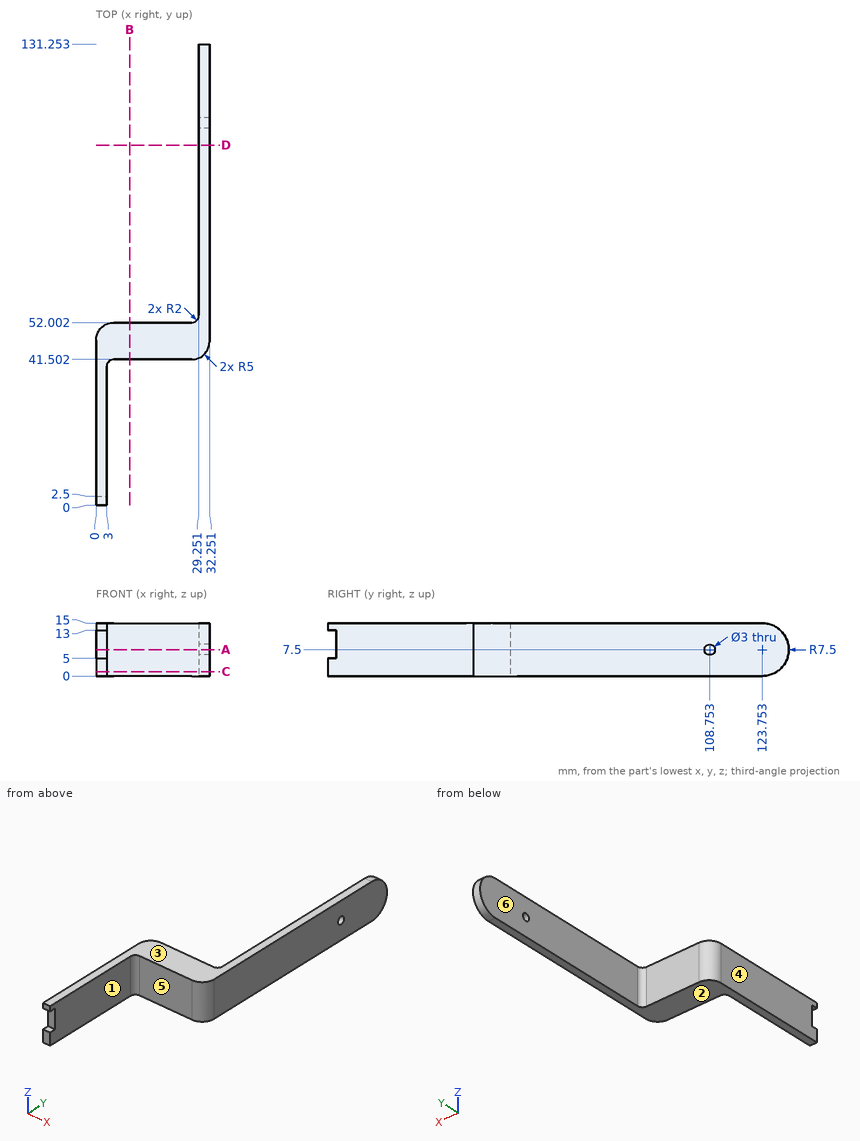
The figure shows three views and two pictorial views of one solid part (mm, origin at its lowest corner). Answer the questions. A direction names the side the tool comes from. Coordinates: 2 decimals unless noted, no trailing zeros. Write each loop counter-clockwise with the first axis right and the second up, starting at its lowest first coordinate (ties: lowest second). Pieces come first, ordered by that corner, then holes. Notation, with made-up numbers: (52, 76.5) -> (59, 76.5) arc R26 ccw to (59, 106.5) -> close; hole circle Ø8 at (0.5, 71.5). An arc over 180 degrees is marked (long way). Return JSON: item names as keys, results as strings.
(1) The part is cut by section A-A on z = 7.5. Give the vertices of the cut face in (x, y).
Answers below:
{"outline": "(0, 2.5) -> (3, 2.5) -> (3, 39.5) arc R2 cw to (5, 41.5) -> (27.25, 41.5) arc R5 ccw to (32.25, 46.5) -> (32.25, 107.25) -> (29.25, 107.25) -> (29.25, 54) arc R2 cw to (27.25, 52) -> (5, 52) arc R5 ccw to (0, 47) -> close; (29.25, 110.25) -> (32.25, 110.25) -> (32.25, 131.25) -> (29.25, 131.25) -> close"}
(2) The part is cut by section C-C on z = 1.25. Give the vertices of the cut face in (x, y), then the cut area to 3 significant figures.
Answers below:
{"outline": "(0, 0) -> (3, 0) -> (3, 39.5) arc R2 cw to (5, 41.5) -> (27.25, 41.5) arc R5 ccw to (32.25, 46.5) -> (32.25, 127.9) -> (29.25, 127.9) -> (29.25, 54) arc R2 cw to (27.25, 52) -> (5, 52) arc R5 ccw to (0, 47) -> close", "area": "682 mm^2"}
(3) Which of the six approach directions +Z, -Z, +X, -X, +Y, -Y give full straight-line access (tool end or side, diameter ignored) to the marked faces 4, 5 and 6?
Answers below:
{"face 4": "+Z, -Z, -X, +Y, -Y", "face 5": "+Z, -Z, +X, -Y", "face 6": "+Z, -Z, -X, +Y"}
(4) Each of these flat-tipped pins is pushed along its axis until it touches: P1, Ø3, axis at x = 21, z = 6, coming from the -Y side; P2, Ø7.5, axis at x = 13, z = 7.5, coming from the +Y side; P3, Ø1, axis at y = 49.5, z = 8, coming from the -X side. Where does it stop, or does it pass through?
Answers below:
{"P1": "y = 41.5", "P2": "y = 52", "P3": "x = 0.42"}
(5) The part is cut by section B-B on x = 9.5. Give the vertices of the cut face in (y, z), then the cut area to 4 significant figures.
Answers below:
{"outline": "(41.5, 0) -> (52, 0) -> (52, 15) -> (41.5, 15) -> close", "area": "157.5 mm^2"}
(6) For a pull along Z with two mould halves and no side action, classify the marked faces 1, 2 and 3 as pulls with the +Z half, pulls with the -Z half, needs draft (parallel to the pull), parting line crosses it, or undercut.
Answers below:
{"face 1": "needs draft", "face 2": "pulls with the -Z half", "face 3": "pulls with the +Z half"}
(7) The part is cut by section D-D on y = 102.5. Give the vertices of the cut face in (x, z), then the cut area to 3 significant figures.
Answers below:
{"outline": "(29.25, 0) -> (32.25, 0) -> (32.25, 15) -> (29.25, 15) -> close", "area": "45.0 mm^2"}
(8) Consider line 1 along X through (y, z) = (14, 4.25); line 2 along X through (y, z) = (115, 4); line 3 along Y through (x, z) = (30.8, 7.5) (1 decimal). Determine where each line is inside the solid, lowest interval first. Write a range as from..to.
Answers below:
{"line 1": "0..3", "line 2": "29.25..32.25", "line 3": "43..107.3, 110.3..131.3"}
